Input: dimensioned drawing with shaded views. Units: mm. Origin: part minimum x, y, z. A direction names the side the tool comes from. Coordinates: 2 decimals unless noted, no trailing zeros. Write each loop counter-clockwise with the first axis right and the second up, starting at its lowest first coordinate (ties: lowest second). Pieces come first, ordered by that corner, then holes. Notation, with made-up numbers: (-40, -16) -> (-12, -16) arc R13 cw to (-12, 8) -> close; hole circle Ø11 at (-0.5, -31). An arc over 180 degrees is marked (long way). One line per item, written item: value. Start each with the question number.
1. Section query A-A, the plane x = 19. Output: boundary loops of the cut face in (y, z).
2. Section query D-D, the plane y = 31.5. Output: boundary loops of the cut face in (x, z).
3. Access query for the marked faces 1 and 2. Directions: +Z, -Z, +X, -X, +Y, -Y. A direction counts if a zero-diameter tool reaches every point of the face in a straight line with its end or side. Return the directions, or none.
4. Line query: line 1 (Y direction, x = 19, z = 1.7); line 2 (Y direction, x = 19, z = 14.5); line 3 (X direction, y = 30.5, z = 16.75). Output: solid intervals per line, ascending.
5. Section query C-C, the plane z = 5.25. Output: boundary loops of the cut face in (x, y), and give its area (3 significant figures).
6. Mould query, pull axis Y, two halves, no side actions, for the marked faces 3, 4 and 5. Classes: released by +Y, released by -Y, zero draft, split by the parting line, or undercut.
7. First-contact query: P1, Ø4, axis at y = 9.5, z = 13, coming from the -X side; P2, Ø8, axis at x = 32, z = 17.5, coming from the +Y side; P3, Ø3, axis at x = 33.5, z = 9.5, coming from the -Y side; P4, Ø5, axis at x = 32.5, y = 25, coming from the -Z side. Flat tips, straight axial feed; report the tip coordinate or a pass-through.
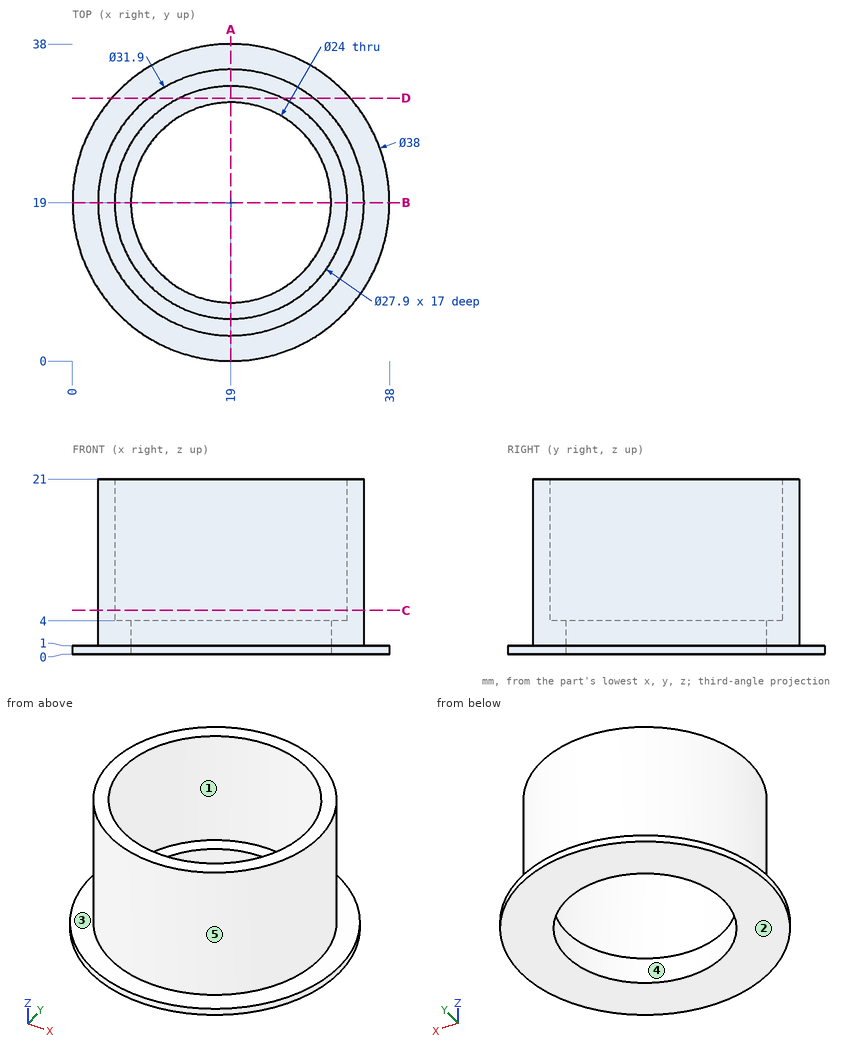
Computed values:
1. outline: (0, 0) -> (7, 0) -> (7, 4) -> (5.05, 4) -> (5.05, 21) -> (3.05, 21) -> (3.05, 1) -> (0, 1) -> close; (31, 0) -> (38, 0) -> (38, 1) -> (34.95, 1) -> (34.95, 21) -> (32.95, 21) -> (32.95, 4) -> (31, 4) -> close
2. outline: (4.69, 0) -> (33.31, 0) -> (33.31, 1) -> (28.91, 1) -> (28.91, 21) -> (25.19, 21) -> (25.19, 4) -> (12.81, 4) -> (12.81, 21) -> (9.09, 21) -> (9.09, 1) -> (4.69, 1) -> close
3. face 1: +Z
3. face 2: -Z, +X, -X, +Y, -Y
4. line 1: y = 3.05 to 7, 31 to 34.95
4. line 2: y = 3.05 to 5.05, 32.95 to 34.95
4. line 3: x = 7.95 to 11.1, 26.9 to 30.05
5. outline: circle Ø31.9 at (19, 19); hole circle Ø27.9 at (19, 19)
5. area: 188 mm²
6. face 3: zero draft
6. face 4: undercut
6. face 5: split by the parting line
7. P1: stops at x = 4.92
7. P2: stops at y = 32.17
7. P3: stops at y = 9.76
7. P4: stops at z = 0
